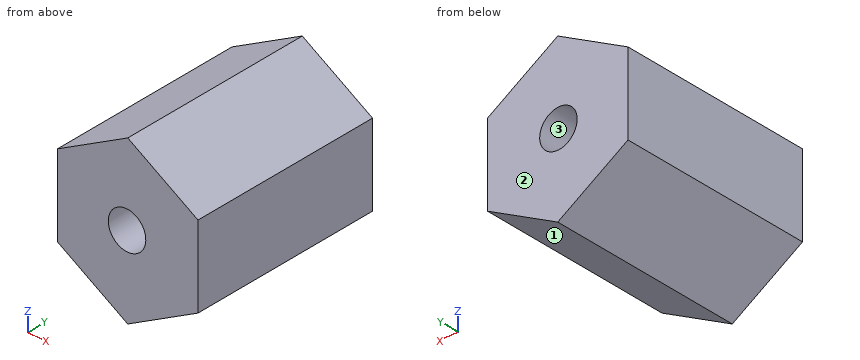
Autodesk Fusion 360 part; units mm, degrees
sketch "Sketch1" plane through (0, 0, 0) normal (0, 1, 0) x (1, 0, 0)
  line L0 (3.75, 2.1651) -> (0, 4.3301)
  line L1 (0, 4.3301) -> (-3.75, 2.1651)
  line L2 (-3.75, 2.1651) -> (-3.75, -2.1651)
  line L3 (-3.75, -2.1651) -> (0, -4.3301)
  line L4 (0, -4.3301) -> (3.75, -2.1651)
  line L5 (3.75, -2.1651) -> (3.75, 2.1651)
  dimension "d4" = 3.75
extrude "Extrude1" add sketch "Sketch1" along normal blind 10
hole "Hole1" at (-0.0367, 0, 0.0102) direction (0, 1, 0) diameter 2 depth 10 tip angle 180
Part model, mm, in its own coordinate system. Face numbers are marked on the shaded views. Give positions to 0.01 mm unless a question says otherwise; leave off trailing zeros. Order: outer loops, then holes, each group sorted by start corner. A loop starts at its lowest first (then second) coordinate and runs counter-clockwise, first axis right, second up. Notation, with made-up numbers: (73.25, -0.5) -> (80.25, -0.5) arc R27 ccw to (80.25, 15.5) -> close; hole circle Ø3 at (17.5, 46). An arc over 180 degrees is marked (long way). Use one line per item in the form item = value.
(1) Saw through at D-D (x = 2.5). Write the cut outline in (y, z).
Solution:
outline = (0, -2.89) -> (10, -2.89) -> (10, 2.89) -> (0, 2.89) -> close
(2) Saw through at B-B (x = -0.25). Write the cut outline in (y, z), then the cut area to 3 significant figures.
Solution:
outline = (0, -4.19) -> (10, -4.19) -> (10, -0.97) -> (0, -0.97) -> close; (0, 0.99) -> (10, 0.99) -> (10, 4.19) -> (0, 4.19) -> close
area = 64.2 mm²
(3) Saw through at C-C (y = 5.75). Write the cut outline in (x, z), then the cut area to 3 significant figures.
Solution:
outline = (-3.75, -2.17) -> (0, -4.33) -> (3.75, -2.17) -> (3.75, 2.17) -> (0, 4.33) -> (-3.75, 2.17) -> close; hole circle Ø2 at (-0.04, 0.01)
area = 45.6 mm²
(4) Saw through at A-A (z = 0.5). Write the cut outline in (x, y), then the cut area to 3 significant figures.
Solution:
outline = (-3.75, 0) -> (-0.91, 0) -> (-0.91, 10) -> (-3.75, 10) -> close; (0.84, 0) -> (3.75, 0) -> (3.75, 10) -> (0.84, 10) -> close
area = 57.6 mm²
(5) Flat gauge pins, fed straight in: P1, Ø1.5, axis at x = 1, y = 3, coming from the +Z side; P2, Ø1.5, axis at x = 0.5, y = 2, coming from the -Z side. Where does each tip first touch, or does it go through?
Solution:
P1 = 4.19
P2 = -4.33
(6) Drill centre lines: line 1 (X direction, y = 8.5, z = -0.25); line 2 (Z direction, x = 0.25, y = 7.5); line 3 (Z direction, x = 0.5, y = 2). Where is each one in solid material? Low to high. Write a range as from..to.
Solution:
line_1 = -3.75..-1, 0.93..3.75
line_2 = -4.19..-0.95, 0.97..4.19
line_3 = -4.04..-0.83, 0.85..4.04
(7) Pull direction Z, two halves, no side cores. Call the marked faces 1, 2 and 3: +Z half, -Z half, draft (parallel to the pull), parting line (faces both ways), or undercut.
Solution:
face_1 = -Z half
face_2 = draft
face_3 = undercut
